Verification items for the finished model (mm, model axes). Give positions to 0.01 mm unless a question says otherwise; leave off trailing zeros. Write each loop counter-clockwise with the first axis right and the second up, starting at its lowest first coordinate (ties: lowest second). Pieces come first, ordered by that corner, then holes. Notation, with made-up numbers: M -24,44.25 L 4,44.25 A28 ccw 4,82.25 Z; hole C 22,-35 d10. An arc over 180 degrees is marked long. Answer as a JSON object with one key per item and string values.
```python
from build123d import *

# Parameters (mm, degrees)
SKETCH_1_W           = 90
SKETCH_1_H           = 60
EXTRUDE_1_DEPTH      = 6.5
EXTRUDE_2_DEPTH      = 0.05
EXTRUDE_2_DEPTH_BACK = 6.55
SKETCH_2_W           = 90.2
SKETCH_2_H           = 10.2
SKETCH_3_W           = 0.5
SKETCH_3_H           = 5
EXTRUDE_3_DEPTH      = 6.55
FILLET_1_R           = 2


with BuildPart() as part:
    # Sketch 1 → Extrude 1 (new body)
    with BuildSketch(Plane.XY):
        with Locations((45, 30)):
            Rectangle(SKETCH_1_W, SKETCH_1_H)
    extrude(amount=EXTRUDE_1_DEPTH)

    # Sketch 2 → Extrude 2 (add, two sides: drawn at the far end of the back side and taken through both)
    with BuildSketch(Plane.XY.offset(6.5).offset(-EXTRUDE_2_DEPTH_BACK)):
        with Locations((45, 55)):
            Rectangle(SKETCH_2_W, SKETCH_2_H)
        with Locations((45, 5)):
            Rectangle(SKETCH_2_W, SKETCH_2_H)
    extrude(amount=EXTRUDE_2_DEPTH + EXTRUDE_2_DEPTH_BACK)

    # Sketch 3 → Extrude 3 (add)
    with BuildSketch(Plane(origin=(90, 0, 0), x_dir=(0, 0, -1), z_dir=(1, 0, 0))):
        with Locations((-3.25, 47.4)):
            Rectangle(SKETCH_3_W, SKETCH_3_H)
        with Locations((-3.25, 12.6)):
            Rectangle(SKETCH_3_W, SKETCH_3_H)
    extrude(amount=EXTRUDE_3_DEPTH)

    # Fillet 1
    fillet_1_edges = [part.edges().sort_by_distance(p)[0] for p in [
        (0, 30, 0),
        (90, 30, 0),
        (0, 30, 6.5),
        (90, 30, 6.5),
        (90.1, 55, -0.05),
        (90.1, 60.1, 3.25),
        (45, 60.1, 6.55),
        (-0.1, 60.1, 3.25),
        (-0.1, 55, 6.55),
        (90.1, 55, 6.55),
        (-0.1, 55, -0.05),
        (45, 60.1, -0.05),
        (-0.1, 5, -0.05),
        (-0.1, -0.1, 3.25),
        (45, -0.1, -0.05),
        (90.1, -0.1, 3.25),
        (90.1, 5, 6.55),
        (-0.1, 5, 6.55),
        (45, -0.1, 6.55),
        (90.1, 5, -0.05),
    ]]
    fillet(fillet_1_edges, radius=FILLET_1_R)


solid = part.part
```
1) Section check D-D on y = 26.5. Record the boundary of the cut face in (x, z).
Completed:
{"outline": "M 0,2 A2 ccw 2,0 L 88,0 A2 ccw 90,2 L 90,4.5 A2 ccw 88,6.5 L 2,6.5 A2 ccw 0,4.5 Z"}
2) Section check A-A on y = 47.5. Record the boundary of the cut face in (x, z).
Completed:
{"outline": "M 0,2 A2 ccw 2,0 L 88,0 A2 ccw 90,2 L 90,3 L 96.55,3 L 96.55,3.5 L 90,3.5 L 90,4.5 A2 ccw 88,6.5 L 2,6.5 A2 ccw 0,4.5 Z"}
3) Go/stop test with flat-tipped pins: pin 1 (3 mm diameter, centred on x = 12.5, y = 12, fed in from -Z); pin 2 (1.3 mm diameter, centred on y = 8, z = 3.5, fed in from +X); pin 3 (0.6 mm diameter, centred on x = 95, z = 3.5, fed in from +Y); pin 4 (3 mm diameter, centred on x = 60.5, z = 5, fed in from -Y). Record where each tip stops, or that it passes through.
Completed:
{"pin 1": "stops at z = 0", "pin 2": "stops at x = 90.1", "pin 3": "stops at y = 49.9", "pin 4": "stops at y = -0.1"}
4) Thickness scan on L1, parallel to Y at x = 67, z = 4.75; L2, parallel to Z at x = 11.5, y = 20; L3, parallel to X at y = 37, z = 2. Record the ranges inside material, lowest first.
Completed:
{"L1": "y = -0.09 to 60.09", "L2": "z = 0 to 6.5", "L3": "x = 0 to 90"}
5) Section check C-C on y = 7. Record the boundary of the cut face in (x, z), and give its area (3 significant figures).
Completed:
{"outline": "M -0.1,1.95 A2 ccw 1.9,-0.05 L 88.1,-0.05 A2 ccw 90.1,1.95 L 90.1,4.55 A2 ccw 88.1,6.55 L 1.9,6.55 A2 ccw -0.1,4.55 Z", "area": "592 mm2"}
6) Section check B-B on x = 26. Record the boundary of the cut face in (y, z), and give its area (3 significant figures).
Completed:
{"outline": "M -0.1,1.95 A2 ccw 1.9,-0.05 L 10.1,-0.05 L 10.1,0 L 49.9,0 L 49.9,-0.05 L 58.1,-0.05 A2 ccw 60.1,1.95 L 60.1,4.55 A2 ccw 58.1,6.55 L 49.9,6.55 L 49.9,6.5 L 10.1,6.5 L 10.1,6.55 L 1.9,6.55 A2 ccw -0.1,4.55 Z", "area": "390 mm2"}
7) Release check for a two-part mould opening along Y. For faces 1 (the face through (-0.1, 6, 3)), 2 (the face through (45.6, 0.5, 5.98)), 3 (the face through (89.43, 30.28, 5.9)) record: pulls with the +Y half, pulls with the -Y half, needs draft (parallel to the pull), parting line crosses it, or undercut.
Completed:
{"face 1": "needs draft", "face 2": "pulls with the -Y half", "face 3": "undercut"}
